Read the model definition and answer for the solid it produces. Units are mm, in the model's axes. A direction names the side the tool comes from. Coordinates: 2 decimals unless noted, no trailing zeros. Write each loop counter-clockwise with the first axis right and the second up, starting at its lowest first coordinate (ties: lowest second). Pieces come first, ordered by that corner, then holes.
(1) Section C-C on x = -7 is taken. Write down the section's boundary in (y, z).
(2) Section D-D on y = -3.75 is taken. Write down the section's boundary in (x, z), then the cut area to 3 significant figures.
(3) Section A-A on z = 1.5 is taken. Write down the section's boundary in (x, y).
(4) Which of the six approach directions +Z, -Z, +X, -X, +Y, -Y give full straight-line access (tool end or side, diameter ignored) to faces 4 (the flat face through (0, -7.5, 3)), 5 (the cylindrical face through (25.43, -6.9, 3.48)), 6 (the cylindrical face through (-25.4, -6.93, 3.48)), 7 (the flat face through (26, 0, 3)), 8 (the cylindrical face through (25.4, 6.93, 3.48))?
(5) Section B-B on y = -0.5 is taken. Write down the section's boundary in (x, z).
(6) The mould has two halves that part along Y. Classify faces 1 (the cylindrical face through (26.43, 8.4, 1.49)), 2 (the cylindrical face through (13.195, -4.295, 2.465)), 3 (the flat face through (-0.3, -9, 1.5)): +Y half, -Y half, draft (parallel to the pull), parting line (faces both ways), or undercut.
(7) Given pin 1 (0.9 mm diameter, centred on x = -3, z = 3, fed in from -Y); pin 2 (0.9 mm diameter, centred on y = 1.5, z = 3.5, fed in from -X); pin 3 (4 mm diameter, centred on x = 14.63, y = -4.75, fed in from -Z); pin 4 (0.9 mm diameter, centred on x = 2.5, z = 4, fed in from +Y), each flat-ended and moving along its own axis, determine where each tip first touches the part or whether it passes through.
(8) Find the intervals of material crossed by probe 1 along Y at (x, z) = (4.5, 0.85); probe 2 along X at (y, z) = (-4.25, 1.3); probe 3 along X at (y, z) = (-4.75, 0.8), in increasing order.
from build123d import *

# Parameters (mm, degrees)
BOSS_EXTRUDE1_DEPTH = 2
BOSS_EXTRUDE2_DEPTH = 3
SKETCH4_R           = 1.5
CUT_EXTRUDE1_DEPTH  = 7
FILLET1_R           = 1


with BuildPart() as part:
    # Sketch1 → Boss-Extrude1 (new body)
    with BuildSketch(Plane.XY):
        with BuildLine():
            Line((25, 9), (-25, 9))
            ThreePointArc((-25, 9), (-26.414213562, 8.414213562), (-27, 7))
            Line((-27, 7), (-27, -7))
            ThreePointArc((-27, -7), (-26.414213562, -8.414213562), (-25, -9))
            Line((-25, -9), (25, -9))
            ThreePointArc((25, -9), (26.414213562, -8.414213562), (27, -7))
            Line((27, -7), (27, 7))
            ThreePointArc((27, 7), (26.414213562, 8.414213562), (25, 9))
        make_face()
    extrude(amount=BOSS_EXTRUDE1_DEPTH)

    # Sketch2 → Boss-Extrude2 (add)
    with BuildSketch(Plane.XY.offset(2)):
        with BuildLine():
            Line((24, -7.5), (-24, -7.5))
            ThreePointArc((-24, -7.5), (-25.414213562, -6.914213562), (-26, -5.5))
            Line((-26, -5.5), (-26, 5.5))
            ThreePointArc((-26, 5.5), (-25.414213562, 6.914213562), (-24, 7.5))
            Line((-24, 7.5), (24, 7.5))
            ThreePointArc((24, 7.5), (25.414213562, 6.914213562), (26, 5.5))
            Line((26, 5.5), (26, -5.5))
            ThreePointArc((26, -5.5), (25.414213562, -6.914213562), (24, -7.5))
        make_face()
    extrude(amount=BOSS_EXTRUDE2_DEPTH)

    # Sketch4 → Cut-Extrude1 (cut)
    with BuildSketch(Plane(origin=(0, 0, 0), x_dir=(-1, 0, 0), z_dir=(0, 0, -1))):
        with Locations((-20.625599185, -4.74532022)):
            Circle(SKETCH4_R)
        with Locations((-14.625599185, -4.74532022)):
            Circle(SKETCH4_R)
    extrude(amount=-CUT_EXTRUDE1_DEPTH, mode=Mode.SUBTRACT)

    # Fillet1
    fillet1_edges = [part.edges().sort_by_distance(p)[0] for p in [
        (0, -9, 0),
        (-26.414213562, -8.414213562, 0),
        (-27, 0, 0),
        (-26.414213562, 8.414213562, 0),
        (0, 9, 0),
        (26.414213562, 8.414213562, 0),
        (27, 0, 0),
        (26.414213562, -8.414213562, 0),
    ]]
    fillet(fillet1_edges, radius=FILLET1_R)


solid = part.part
Response:
1. outline: (-9, 1) arc R1 ccw to (-8, 0) - (8, 0) arc R1 ccw to (9, 1) - (9, 2) - (7.5, 2) - (7.5, 5) - (-7.5, 5) - (-7.5, 2) - (-9, 2) - close
2. outline: (-27, 1) arc R1 ccw to (-26, 0) - (13.5, 0) - (13.5, 5) - (-26, 5) - (-26, 2) - (-27, 2) - close; (15.75, 0) - (19.5, 0) - (19.5, 5) - (15.75, 5) - close; (21.75, 0) - (26, 0) arc R1 ccw to (27, 1) - (27, 2) - (26, 2) - (26, 5) - (21.75, 5) - close
2. area: 241 mm2
3. outline: (-27, -7) arc R2 ccw to (-25, -9) - (25, -9) arc R2 ccw to (27, -7) - (27, 7) arc R2 ccw to (25, 9) - (-25, 9) arc R2 ccw to (-27, 7) - close; hole circle Ø3 at (14.63, -4.75); hole circle Ø3 at (20.63, -4.75)
4. face 4: +Z, +X, -X, -Y
4. face 5: +Z, +X, -Y
4. face 6: +Z, -X, -Y
4. face 7: +Z, +X, +Y, -Y
4. face 8: +Z, +X, +Y
5. outline: (-27, 1) arc R1 ccw to (-26, 0) - (26, 0) arc R1 ccw to (27, 1) - (27, 2) - (26, 2) - (26, 5) - (-26, 5) - (-26, 2) - (-27, 2) - close
6. face 1: +Y half
6. face 2: undercut
6. face 3: -Y half
7. pin 1: stops at y = -7.5
7. pin 2: stops at x = -26
7. pin 3: stops at z = 0
7. pin 4: stops at y = 7.5
8. probe 1: y = -8.99 to 8.99
8. probe 2: x = -27 to 13.21, 16.04 to 19.21, 22.04 to 27
8. probe 3: x = -26.98 to 13.13, 16.13 to 19.13, 22.13 to 26.98
